Work out the finished part from the listing and answer in its coordinate system (mm). Face numbers are marked on the shaded views. A direction names the side the tool comes from. Coordinates: 2 decimals unless noted, no trailing zeros. Order: outer loops, then holes, each group sorted by start corner. A loop starts at its lowest first (then second) coordinate and runs counter-clockwise, first axis right, second up. Notation, with made-up numbers: M -17,-19 L 4,-19 A25 ccw 4,5 Z; hole C 23,51 d2. An arc over 180 degrees is marked long. Use a Markdown table: item, result.
from build123d import *

# Parameters (mm, degrees)
F2_SIZE2 = 0.05
F2_SIZE  = 0.05


with BuildPart() as f1:
    # F0 (on Front) → F1 (revolve)
    with BuildSketch(Plane.XZ):
        Polygon((0, 4), (0, 2.5), (10, 2.5), (10, 5), (8, 5), (8, 4), align=None)
    revolve(axis=Axis((5, 0, 0), (1, 0, 0)))

    # F2
    f2_edges = [f1.edges().sort_by_distance(p)[0] for p in [
        (10, 0, -5),
        (8, 0, -5),
    ]]
    chamfer(f2_edges, length=F2_SIZE, length2=F2_SIZE2)


solid = f1.part
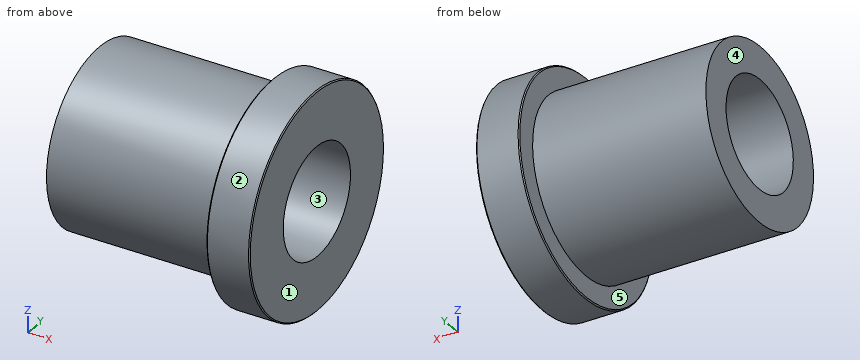
1. Section A-A on z = 0 is taken. Determine the outline of the cut face in (x, y).
Answers below:
| item | result |
|---|---|
| outline | M 0,-4 L 8,-4 L 8,-4.95 L 8.05,-5 L 9.95,-5 L 10,-4.95 L 10,-2.5 L 0,-2.5 Z; M 0,2.5 L 10,2.5 L 10,4.95 L 9.95,5 L 8.05,5 L 8,4.95 L 8,4 L 0,4 Z |
2. For the marked faces 4 and 5, determine the directions among +Z, -Z, +X, -X, +Y, -Y from which every point of the face is accessible in a straight line to the end or side of a thin tool.
Answers below:
| item | result |
|---|---|
| face 4 | +Z, -Z, -X, +Y, -Y |
| face 5 | -X |
3. Find the intervals of material crossed by probe 1 along Y at (x, z) = (4.5, 0); probe 2 along Z at (x, y) = (8.25, 2.25), in increasing order.
Answers below:
| item | result |
|---|---|
| probe 1 | -4 to -2.5, 2.5 to 4 |
| probe 2 | -4.47 to -1.09, 1.09 to 4.47 |
4. Flat-ended cylindrical pins translate along their axes: P1, Ø4, axis at x = 3, y = 1.5, coming from the -Z side; P2, Ø5, axis at x = 7, z = 2.5, coming from the +Y side. Find the tip coordinate at first contact, or state that the pin passes through.
Answers below:
| item | result |
|---|---|
| P1 | z = -4 |
| P2 | y = 4.99 |
5. For a pull along Z with two mould halves and no side action, classify the marked faces 1, 2 and 3 as +Z half, -Z half, draft (parallel to the pull), parting line (faces both ways), or undercut.
Answers below:
| item | result |
|---|---|
| face 1 | draft |
| face 2 | parting line |
| face 3 | undercut |
6. Section C-C on x = 8.5 is taken. Determine the outline of the cut face in (y, z), then the cut area to 3 significant figures.
Answers below:
| item | result |
|---|---|
| outline | C 0,0 d10; hole C 0,0 d5 |
| area | 58.9 mm² |
7. Section D-D on x = 3.75 is taken. Determine the outline of the cut face in (y, z).
Answers below:
| item | result |
|---|---|
| outline | C 0,0 d8; hole C 0,0 d5 |
